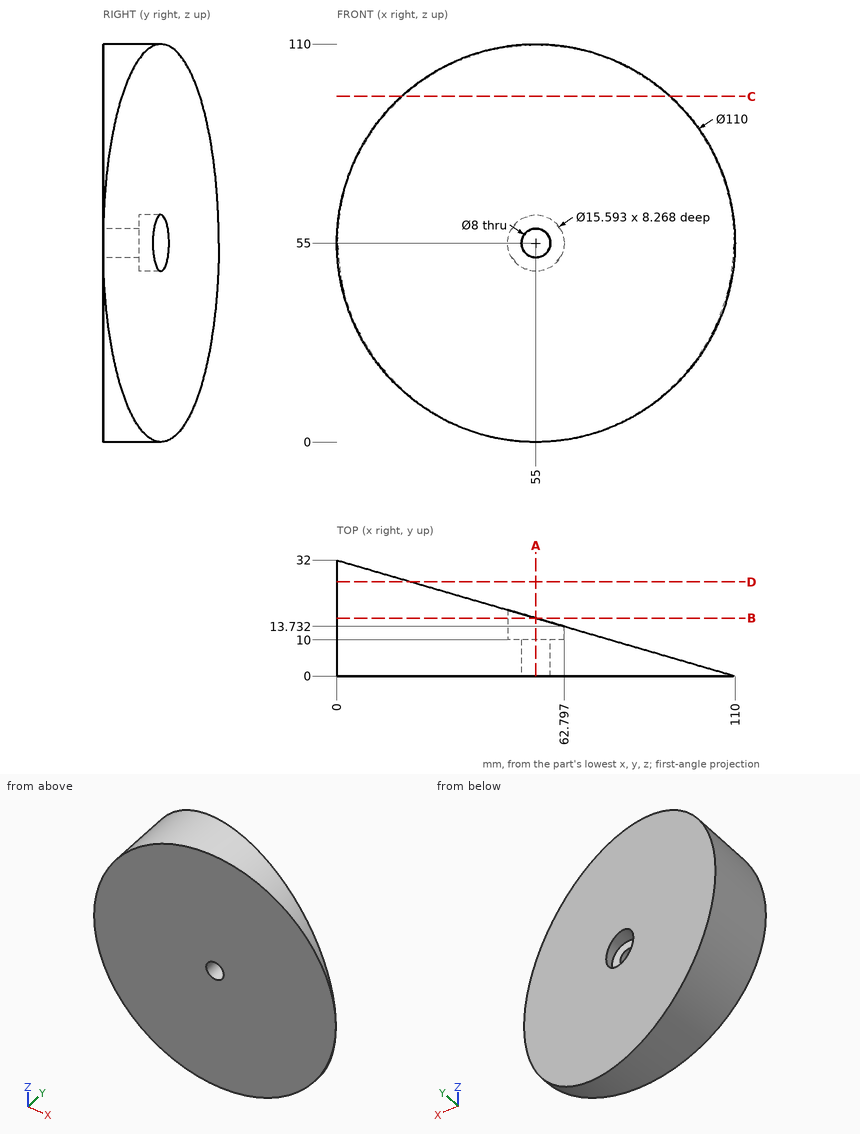
Check sheet for the drawn part. Datum: minimum x, y, z corner. Units: mm. Give positions to 0.01 mm unless a question says otherwise; leave off trailing zeros. Write each loop counter-clockwise with the first axis right and the second up, starting at its lowest first coordinate (ties: lowest second). Pieces come first, ordered by that corner, then holes. Notation, with made-up numbers: (81, 79) -> (116, 79) arc R5 cw to (116, 88) -> close; hole circle Ø2 at (86.25, 84.25). An arc over 180 degrees is marked (long way). Use one line per item in the form item = value. Start each with the question number.
1. Section check C-C (z = 95.5). Record the cut outline in (x, y) (1 decimal), and give its area (3 significant figures).
2. Section check D-D (y = 26). Record the cut outline in (x, z) (1 decimal), and give its area (3 significant figures).
3. Section check B-B (y = 16). Record the cut outline in (x, z), and give its area (3 significant figures).
4. Section check A-A (x = 55). Record the cut outline in (y, z), and give its area (3 significant figures).
5. Thickness scan on line 1 along Z through (x, y) = (55, 12); line 2 along Z through (x, y) = (55, 6.25); line 3 along Y through (x, z) = (47.5, 53). Record the ranges inside material, lowest first. Write a range as from..to.
6. Go/stop test with flat-tipped pins: P1, Ø5, axis at x = 75.5, z = 85.5, coming from the +Y side; P2, Ø8, axis at x = 33.5, y = 20.5, coming from the +Z side; P3, Ø5, axis at x = 55, z = 49.5, coming from the -Y side; P4, Ø6, axis at x = 13.5, y = 3.5, coming from the -Z side. Record where each tip stops, or that it passes through.
Conclusion:
q1.outline = (17.8, 0) -> (92.2, 0) -> (92.2, 5.2) -> (17.8, 26.8) -> close
q1.area = 1,190 mm²
q2.outline = (20.6, 12.1) -> (20.6, 97.9) arc R55 ccw to start
q2.area = 1,230 mm²
q3.outline = (55, 0) -> (55, 47.2) arc R7.8 cw to (55, 62.8) -> (55, 110) arc R55 ccw to start
q3.area = 4,660 mm²
q4.outline = (0, 0) -> (16, 0) -> (16, 47.2) -> (10, 47.2) -> (10, 51) -> (0, 51) -> close; (0, 59) -> (10, 59) -> (10, 62.8) -> (16, 62.8) -> (16, 110) -> (0, 110) -> close
q4.area = 1,590 mm²
q5.line_1 = 0..47.2, 62.8..110
q5.line_2 = 0..51, 59..110
q5.line_3 = 0..10
q6.P1 = 10.76
q6.P2 = 107.14
q6.P3 = 0
q6.P4 = 15.72
